Source: CAD feature listing. Evaluate the final solid. Frame: model axes, mm. Face numbers are marked on the shaded views. Coordinates: 2 decimals unless noted, no trailing zeros. Answer as CSV lines item,"result". Start each with the question number.
1. Line query: probe 1 along Z at (x, y) = (-98, -10); probe 2 along Z at (x, y) = (-97.5, -16.5); probe 3 along Z at (x, y) = (-45, -15.25). Output: solid intervals per line, ascending. Write a range as [from, to].
2. Mould query, pull axis Z, two halves, no side actions, for the marked faces 1, 2 and 3. Classes: pulls with the +Z half, pulls with the -Z half, needs draft (parallel to the pull), parting line crosses it, or undercut.
3. Contact query for flat-ended pins moving along their axis: pin 1 Ø12 at (x, z) = (-98.5, 41.5) entering from +Y; pin 2 Ø1 at (x, z) = (-86.5, 88) entering from -Y. Output: stop coordinate, or through.
4. Section A-A on y = -11.25. Count the separate pieces of the cut face and the enclosed holes in it, plus the area to 3 significant figures.
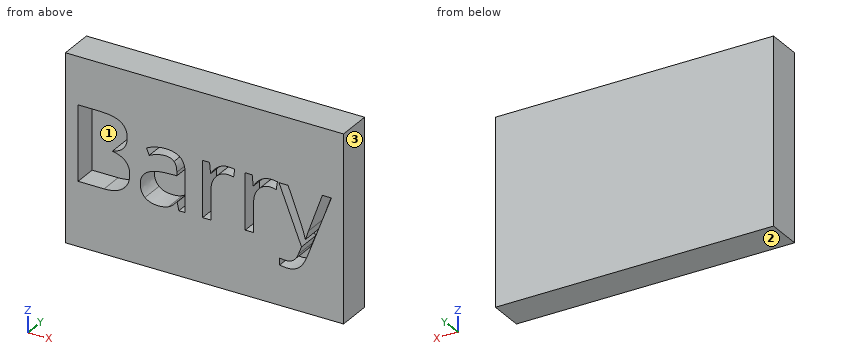
```python
from build123d import *

# Parameters (mm, degrees)
F0_W     = 152.4
F0_H     = 101.6
F1_DEPTH = 6.35
F2_W     = 152.4
F2_H     = 101.6
F3_DEPTH = 12.7


with BuildPart() as f1:
    # F0 (on Front) → F1 (new body)
    with BuildSketch(Plane.XZ):
        with Locations((-73.2831337214, 78.9085992667)):
            Rectangle(F0_W, F0_H)
    extrude(amount=F1_DEPTH)

    # F2 (on face) → F3 (join)
    with BuildSketch(Plane.XZ.offset(6.35)):
        with Locations((-73.2831337214, 78.9085992667)):
            Rectangle(F2_W, F2_H)
        with BuildLine():
            Line((-83.8709204292, 62.9637678441), (-87.3141177383, 62.9637678441))
            Line((-87.3141177383, 62.9637678441), (-88.2352848107, 67.3281322256))
            Line((-88.2352848107, 67.3281322256), (-88.4588690515, 67.3281322256))
            add(Edge.make_bspline(
                [(-88.4588690515, 67.3281322256), (-90.7483716779, 64.4483672034), (-93.0244592498, 63.4243513802)],
                knots=[0, 0, 0, 1, 1, 1], degree=2))
            add(Edge.make_bspline(
                [(-93.0244592498, 63.4243513802), (-95.3005468216, 62.4003355571), (-98.7169140219, 62.4003355571)],
                knots=[0, 0, 0, 1, 1, 1], degree=2))
            add(Edge.make_bspline(
                [(-98.7169140219, 62.4003355571), (-103.2690891657, 62.4003355571), (-105.85372299, 64.7524417709)],
                knots=[0, 0, 0, 1, 1, 1], degree=2))
            add(Edge.make_bspline(
                [(-105.85372299, 64.7524417709), (-108.4383568142, 67.1045479847), (-108.4383568142, 71.4331388876)],
                knots=[0, 0, 0, 1, 1, 1], degree=2))
            add(Edge.make_bspline(
                [(-108.4383568142, 71.4331388876), (-108.4383568142, 80.7074131983), (-93.6013065912, 81.15458168)],
                knots=[0, 0, 0, 1, 1, 1], degree=2))
            Line((-93.6013065912, 81.15458168), (-88.4052088337, 81.324505703))
            Line((-88.4052088337, 81.324505703), (-88.4052088337, 83.2294434351))
            add(Edge.make_bspline(
                [(-88.4052088337, 83.2294434351), (-88.4052088337, 86.8336213977), (-89.9524117804, 88.5507483674)],
                knots=[0, 0, 0, 1, 1, 1], degree=2))
            add(Edge.make_bspline(
                [(-89.9524117804, 88.5507483674), (-91.4996147271, 90.2678753372), (-94.9159819274, 90.2678753372)],
                knots=[0, 0, 0, 1, 1, 1], degree=2))
            add(Edge.make_bspline(
                [(-94.9159819274, 90.2678753372), (-98.7437441308, 90.2678753372), (-103.5731637332, 87.924712493)],
                knots=[0, 0, 0, 1, 1, 1], degree=2))
            Line((-103.5731637332, 87.924712493), (-105.0041028747, 91.4752302378))
            add(Edge.make_bspline(
                [(-105.0041028747, 91.4752302378), (-102.7414303573, 92.7004718777), (-100.0450044126, 93.3980547091)],
                knots=[0, 0, 0, 1, 1, 1], degree=2))
            add(Edge.make_bspline(
                [(-100.0450044126, 93.3980547091), (-97.3485784679, 94.0956375406), (-94.6297940991, 94.0956375406)],
                knots=[0, 0, 0, 1, 1, 1], degree=2))
            add(Edge.make_bspline(
                [(-94.6297940991, 94.0956375406), (-89.156451883, 94.0956375406), (-86.5136861561, 91.6675126849)],
                knots=[0, 0, 0, 1, 1, 1], degree=2))
            add(Edge.make_bspline(
                [(-86.5136861561, 91.6675126849), (-83.8709204292, 89.2393878293), (-83.8709204292, 83.8733660488)],
                knots=[0, 0, 0, 1, 1, 1], degree=2))
            Line((-83.8709204292, 83.8733660488), (-83.8709204292, 62.9637678441))
        make_face(mode=Mode.SUBTRACT)
        with BuildLine():
            add(Edge.make_bspline(
                [(-65.6264463755, 92.5350195394), (-63.2206799439, 94.158241128), (-60.3409149217, 94.158241128)],
                knots=[0, 0, 0, 1, 1, 1], degree=2))
            add(Edge.make_bspline(
                [(-60.3409149217, 94.158241128), (-58.3018266451, 94.158241128), (-56.6830767413, 93.818393082)],
                knots=[0, 0, 0, 1, 1, 1], degree=2))
            Line((-56.6830767413, 93.818393082), (-57.326999355, 89.5166322879))
            add(Edge.make_bspline(
                [(-57.326999355, 89.5166322879), (-59.2229937174, 89.9369706607), (-60.6807629678, 89.9369706607)],
                knots=[0, 0, 0, 1, 1, 1], degree=2))
            add(Edge.make_bspline(
                [(-60.6807629678, 89.9369706607), (-64.4012047356, 89.9369706607), (-67.0394987777, 86.9185834092)],
                knots=[0, 0, 0, 1, 1, 1], degree=2))
            add(Edge.make_bspline(
                [(-67.0394987777, 86.9185834092), (-69.6777928198, 83.9001961577), (-69.6777928198, 79.4016812317)],
                knots=[0, 0, 0, 1, 1, 1], degree=2))
            Line((-69.6777928198, 79.4016812317), (-69.6777928198, 62.9637678441))
            Line((-69.6777928198, 62.9637678441), (-74.3194016599, 62.9637678441))
            Line((-74.3194016599, 62.9637678441), (-74.3194016599, 93.5948088411))
            Line((-74.3194016599, 93.5948088411), (-70.4916394565, 93.5948088411))
            Line((-70.4916394565, 93.5948088411), (-69.9550372784, 87.924712493))
            Line((-69.9550372784, 87.924712493), (-69.7314530376, 87.924712493))
            add(Edge.make_bspline(
                [(-69.7314530376, 87.924712493), (-68.0322128071, 90.9117979508), (-65.6264463755, 92.5350195394)],
                knots=[0, 0, 0, 1, 1, 1], degree=2))
        make_face(mode=Mode.SUBTRACT)
        with BuildLine():
            add(Edge.make_bspline(
                [(-42.2574215214, 92.5350195394), (-39.8516550898, 94.158241128), (-36.9718900676, 94.158241128)],
                knots=[0, 0, 0, 1, 1, 1], degree=2))
            add(Edge.make_bspline(
                [(-36.9718900676, 94.158241128), (-34.932801791, 94.158241128), (-33.3140518873, 93.818393082)],
                knots=[0, 0, 0, 1, 1, 1], degree=2))
            Line((-33.3140518873, 93.818393082), (-33.9579745009, 89.5166322879))
            add(Edge.make_bspline(
                [(-33.9579745009, 89.5166322879), (-35.8539688634, 89.9369706607), (-37.3117381137, 89.9369706607)],
                knots=[0, 0, 0, 1, 1, 1], degree=2))
            add(Edge.make_bspline(
                [(-37.3117381137, 89.9369706607), (-41.0321798815, 89.9369706607), (-43.6704739236, 86.9185834092)],
                knots=[0, 0, 0, 1, 1, 1], degree=2))
            add(Edge.make_bspline(
                [(-43.6704739236, 86.9185834092), (-46.3087679657, 83.9001961577), (-46.3087679657, 79.4016812317)],
                knots=[0, 0, 0, 1, 1, 1], degree=2))
            Line((-46.3087679657, 79.4016812317), (-46.3087679657, 62.9637678441))
            Line((-46.3087679657, 62.9637678441), (-50.9503768058, 62.9637678441))
            Line((-50.9503768058, 62.9637678441), (-50.9503768058, 93.5948088411))
            Line((-50.9503768058, 93.5948088411), (-47.1226146024, 93.5948088411))
            Line((-47.1226146024, 93.5948088411), (-46.5860124244, 87.924712493))
            Line((-46.5860124244, 87.924712493), (-46.3624281835, 87.924712493))
            add(Edge.make_bspline(
                [(-46.3624281835, 87.924712493), (-44.663187953, 90.9117979508), (-42.2574215214, 92.5350195394)],
                knots=[0, 0, 0, 1, 1, 1], degree=2))
        make_face(mode=Mode.SUBTRACT)
        with BuildLine():
            Line((-20.0868081983, 62.793843821), (-32.4465450327, 93.5948088411))
            Line((-32.4465450327, 93.5948088411), (-27.4650881465, 93.5948088411))
            Line((-27.4650881465, 93.5948088411), (-20.7575609209, 76.1284079456))
            add(Edge.make_bspline(
                [(-20.7575609209, 76.1284079456), (-18.5574919909, 70.1452936603), (-18.0208898128, 67.489112879)],
                knots=[0, 0, 0, 1, 1, 1], degree=2))
            Line((-18.0208898128, 67.489112879), (-17.797305572, 67.489112879))
            add(Edge.make_bspline(
                [(-17.797305572, 67.489112879), (-17.4395707866, 68.9200520204), (-16.2769327342, 72.3721926992)],
                knots=[0, 0, 0, 1, 1, 1], degree=2))
            add(Edge.make_bspline(
                [(-16.2769327342, 72.3721926992), (-15.1142946817, 75.824333378), (-8.6840119148, 93.5948088411)],
                knots=[0, 0, 0, 1, 1, 1], degree=2))
            Line((-8.6840119148, 93.5948088411), (-3.7114983982, 93.5948088411))
            Line((-3.7114983982, 93.5948088411), (-16.8761384997, 58.7156672679))
            add(Edge.make_bspline(
                [(-16.8761384997, 58.7156672679), (-18.8347364495, 53.5463996193), (-21.4462003827, 51.377632483)],
                knots=[0, 0, 0, 1, 1, 1], degree=2))
            add(Edge.make_bspline(
                [(-21.4462003827, 51.377632483), (-24.0576643159, 49.2088653467), (-27.8585964104, 49.2088653467)],
                knots=[0, 0, 0, 1, 1, 1], degree=2))
            add(Edge.make_bspline(
                [(-27.8585964104, 49.2088653467), (-29.9871183834, 49.2088653467), (-32.0530367688, 49.691807307)],
                knots=[0, 0, 0, 1, 1, 1], degree=2))
            Line((-32.0530367688, 49.691807307), (-32.0530367688, 53.4033057052))
            add(Edge.make_bspline(
                [(-32.0530367688, 53.4033057052), (-30.5147771918, 53.0724010287), (-28.6187828293, 53.0724010287)],
                knots=[0, 0, 0, 1, 1, 1], degree=2))
            add(Edge.make_bspline(
                [(-28.6187828293, 53.0724010287), (-23.834080075, 53.0724010287), (-21.7949917985, 58.4384228092)],
                knots=[0, 0, 0, 1, 1, 1], degree=2))
            Line((-21.7949917985, 58.4384228092), (-20.0868081983, 62.793843821))
        make_face(mode=Mode.SUBTRACT)
        with BuildLine():
            Line((-142.5394252293, 62.9637678441), (-142.5394252293, 103.8260237026))
            Line((-142.5394252293, 103.8260237026), (-130.9935350316, 103.8260237026))
            add(Edge.make_bspline(
                [(-130.9935350316, 103.8260237026), (-122.8640120341, 103.8260237026), (-119.2285322779, 101.3934271621)],
                knots=[0, 0, 0, 1, 1, 1], degree=2))
            add(Edge.make_bspline(
                [(-119.2285322779, 101.3934271621), (-115.5930525216, 98.9608306216), (-115.5930525216, 93.7110726463)],
                knots=[0, 0, 0, 1, 1, 1], degree=2))
            add(Edge.make_bspline(
                [(-115.5930525216, 93.7110726463), (-115.5930525216, 90.0711212052), (-117.6187257437, 87.7100716218)],
                knots=[0, 0, 0, 1, 1, 1], degree=2))
            add(Edge.make_bspline(
                [(-117.6187257437, 87.7100716218), (-119.6443989658, 85.3490220384), (-123.5347647567, 84.6514392069)],
                knots=[0, 0, 0, 1, 1, 1], degree=2))
            Line((-123.5347647567, 84.6514392069), (-123.5347647567, 84.3741947483))
            add(Edge.make_bspline(
                [(-123.5347647567, 84.3741947483), (-114.2247169675, 82.7822749534), (-114.2247169675, 74.5901483685)],
                knots=[0, 0, 0, 1, 1, 1], degree=2))
            add(Edge.make_bspline(
                [(-114.2247169675, 74.5901483685), (-114.2247169675, 69.1168061524), (-117.9272719961, 66.0402869982)],
                knots=[0, 0, 0, 1, 1, 1], degree=2))
            add(Edge.make_bspline(
                [(-117.9272719961, 66.0402869982), (-121.6298270246, 62.9637678441), (-128.2836940324, 62.9637678441)],
                knots=[0, 0, 0, 1, 1, 1], degree=2))
            Line((-128.2836940324, 62.9637678441), (-142.5394252293, 62.9637678441))
        make_face(mode=Mode.SUBTRACT)
    extrude(amount=F3_DEPTH)


solid = f1.part
```
Values:
1,probe 1,"[28.11, 62.41], [80.78, 89.92], [93.83, 129.71]"
1,probe 2,"[28.11, 62.43], [80.85, 90.02], [93.9, 129.71]"
1,probe 3,"[28.11, 85], [89.96, 129.71]"
2,face 1,"undercut"
2,face 2,"pulls with the -Z half"
2,face 3,"needs draft"
3,pin 1,"y = 0"
3,pin 2,"y = -6.35"
4,separate pieces,"1"
4,enclosed holes,"5"
4,area,"13,200 mm²"
